from build123d import *

# Parameters (mm, degrees)
CROQUIS1_R      = 2.15
BOSCHBASE_DEPTH = 235


with BuildPart() as part:
    # Croquis1 → BoschBase (new body)
    with BuildSketch(Plane.XY):
        Polygon((4.4, 0), (0, 0), (0, -0.56736664), (0, -4.4), (0, -4.95), (1.8, -6.75), (1.8, -4.4), (3.410050506, -4.4), (6.175, -7.164949494), (6.175, -12.835050506), (3.410050506, -15.6), (1.8, -15.6), (1.8, -13.25), (0, -15.05), (0, -15.6), (0, -20), (4.4, -20), (4.95, -20), (6.75, -18.2), (4.4, -18.2), (4.4, -16.589949494), (7.164949494, -13.825), (12.835050506, -13.825), (15.6, -16.589949494), (15.6, -18.2), (13.25, -18.2), (15.05, -20), (15.6, -20), (18.2, -20), (20, -20), (20, -15.6), (20, -15.05), (18.2, -13.25), (18.2, -15.6), (16.589949494, -15.6), (13.825, -12.835050506), (13.825, -7.164949494), (16.589949494, -4.4), (18.2, -4.4), (18.2, -6.75), (20, -4.95), (20, -4.4), (20, 0), (15.6, 0), (15.05, 0), (13.25, -1.8), (15.6, -1.8), (15.6, -3.410050506), (12.835050506, -6.175), (7.164949494, -6.175), (4.4, -3.410050506), (4.4, -1.8), (6.75, -1.8), (4.95, 0), align=None)
        with Locations(Location((10, -10, 0), (0, 0, 180))):
            Circle(CROQUIS1_R, mode=Mode.SUBTRACT)
    extrude(amount=BOSCHBASE_DEPTH)


solid = part.part
Geometry check sheet. Reference: the model listing, model coordinates, mm. A direction names the side the tool comes from. Give positions to 0.01 mm unless a question says otherwise; leave off trailing zeros. Order: outer loops, then holes, each group sorted by start corner. A loop starts at its lowest first (then second) coordinate and runs counter-clockwise, first axis right, second up. Notation, with made-up numbers: (1, -7.5) - (15, -7.5) arc R7 cw to (15, -1.5) - close; hole circle Ø6 at (-9.75, -32). An arc over 180 degrees is marked (long way). Use one line per item in the form item = value.
1) Draft check along X on faces 1 (the face through (9.01, -8.09, 115.86)), 2 (the face through (20, -3, 116)), 3 (the face through (18, 0, 116)), 4 (the face through (0, -17, 116)). Enter one of: released by +X, released by -X, zero draft, split by the parting line, or undercut.
Working result:
face_1 = undercut
face_2 = released by +X
face_3 = zero draft
face_4 = released by -X
2) Sectioned sample at A-A (y = -10). Record the boundary of the cut face in (x, z) (3 decimals), and give its area (3 significant figures).
Working result:
outline = (6.175, 0) - (7.85, 0) - (7.85, 235) - (6.175, 235) - close; (12.15, 0) - (13.825, 0) - (13.825, 235) - (12.15, 235) - close
area = 787 mm^2
3) Access from +Z, -Z, +X, -X, +Y, -Y to the whole of each face (thin tool, end or side, straight path). Record for faces 5 (the face through (10, -13.825, 116)), 6 (the face through (10, -6.175, 116)), 7 (the face through (6.175, -10, 116)), 8 (the face through (7.6, -9.9, 0)), 9 (the face through (13.825, -10, 116)).
Working result:
face_5 = +Z, -Z, -Y
face_6 = +Z, -Z, +Y
face_7 = +Z, -Z, -X
face_8 = -Z, +X, -X, +Y, -Y
face_9 = +Z, -Z, +X
4) Material ranges on probe 1 along X at (y, z) = (-10, 84.5) (3 decimals); probe 2 along X at (y, z) = (-5.5, 37); probe 3 along X at (y, z) = (-2, 168), recorded low to high. Write a range as from..to.
Working result:
probe_1 = 6.175..7.85, 12.15..13.825
probe_2 = 0.55..1.8, 4.51..6.49, 13.51..15.49, 18.2..19.45
probe_3 = 0..4.4, 15.6..20
5) Depth check by flat-ended pin: pin 1 Ø6 at (y, z) = (-11, 165) entering from +X; pin 2 Ø5 at (y, z) = (-8.5, 171) entering from -X; pin 3 Ø2 at (y, z) = (-13.5, 100.5) entering from -X. Enter the tip coordinate at first touch or a pass-through.
Working result:
pin_1 = 18.95
pin_2 = 1.05
pin_3 = 0.55
6) Sectioned sample at B-B (x = 10). Record the boundary of the cut face in (y, z) (3 decimals), and give its area (3 significant figures).
Working result:
outline = (-13.825, 0) - (-12.15, 0) - (-12.15, 235) - (-13.825, 235) - close; (-7.85, 0) - (-6.175, 0) - (-6.175, 235) - (-7.85, 235) - close
area = 787 mm^2
